For this review, take the finished solid that the model builds, in its own axes (mm). Face numbers are marked on the shaded views. A direction names the side the tool comes from. Round coordinates to 2 decimals unless told otherwise and drop trailing zeros. Order: outer loops, then holes, each group sorted by start corner. A loop starts at its lowest first (then second) coordinate and runs counter-clockwise, first axis right, second up. Notation, with made-up numbers: M 42,12.25 L 71,12.25 A25 ccw 71,33.25 Z; hole C 0.25,46 d1. An arc over 180 degrees is marked long. Answer as a JSON object with one key per item and string values.
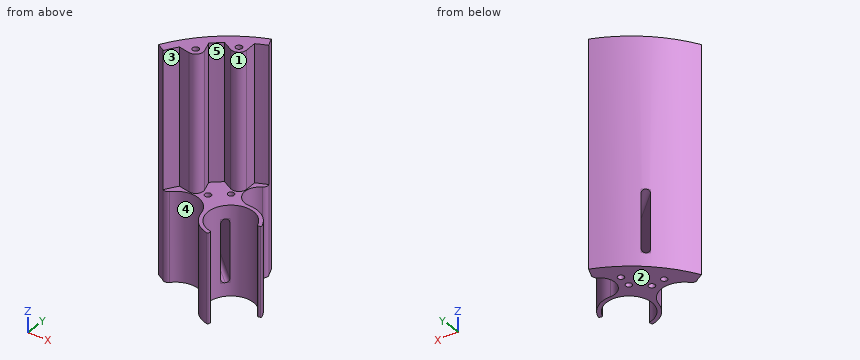
from build123d import *

# Parameters (mm, degrees)
BOSS_EXTRUDE1_DEPTH     = 119
BOSS_EXTRUDE2_DEPTH     = 47
SKETCH4_R               = 1.65
CUT_EXTRUDE1_DEPTH      = 151.148950374
CUT_EXTRUDE2_START      = 44
CUT_EXTRUDE2_DEPTH      = 2.6
BOSS_EXTRUDE3_DEPTH     = 119
SKETCH7_R               = 1.65
CUT_EXTRUDE3_DEPTH      = 151.148950374
CUT_EXTRUDE4_START      = 116
CUT_EXTRUDE4_DEPTH      = 2.6
CUT_EXTRUDE5_START      = 3
CUT_EXTRUDE5_DEPTH      = 2.6
CUT_EXTRUDE_THIN1_DEPTH = 151.148950374
CUT_EXTRUDE6_START      = 7
CUT_EXTRUDE6_DEPTH      = 33
FILLET1_R               = 2


with BuildPart() as part:
    # Sketch1 → Boss-Extrude1 (new body)
    with BuildSketch(Plane(origin=(0, 0, 0), x_dir=(0, 1, 0), z_dir=(0, 0, 1))):
        with BuildLine():
            Line((66.793011614, 25.63943495), (62.125109481, 23.847595202))
            ThreePointArc((62.125109481, 23.847595202), (50.18784505, 43.696878999), (32.170193606, 58.252173078))
            Line((32.170193606, 58.252173078), (34.587369472, 62.629073903))
            ThreePointArc((34.587369472, 62.629073903), (53.95881545, 46.980136869), (66.793011614, 25.63943495))
        make_face()
    extrude(amount=BOSS_EXTRUDE1_DEPTH)

    # Sketch3 → Boss-Extrude2 (add)
    with BuildSketch(Plane(origin=(0, 0, 0), x_dir=(0, 1, 0), z_dir=(0, 0, 1))):
        with BuildLine():
            Line((16.662914887, 22.849921086), (17.643603591, 22.654345869))
            ThreePointArc((17.643603591, 22.654345869), (18.018970735, 22.728818123), (18.231735551, 23.046902612))
            ThreePointArc((18.231735551, 23.046902612), (37.916609506, 29.718164665), (33.851654942, 9.334932723))
            ThreePointArc((33.851654942, 9.334932723), (33.563813587, 9.082754287), (33.538596095, 8.700902631))
            Line((33.538596095, 8.700902631), (33.85956734, 7.753813691))
            ThreePointArc((33.85956734, 7.753813691), (34.111745776, 7.465972336), (34.493597433, 7.440754844))
            ThreePointArc((34.493597433, 7.440754844), (41.448499021, 12.641968592), (43.997873295, 20.944014808))
            ThreePointArc((43.997873295, 20.944014808), (49.930251766, 28.811968202), (58.997685125, 24.954578252))
            ThreePointArc((58.997685125, 24.954578252), (60.351321071, 23.807583941), (62.125109481, 23.847595202))
            ThreePointArc((62.125109481, 23.847595202), (50.18784505, 43.696878999), (32.170193606, 58.252173078))
            ThreePointArc((32.170193606, 58.252173078), (31.867825608, 56.602303211), (32.676329677, 55.132671232))
            ThreePointArc((32.676329677, 55.132671232), (36.307290349, 43.066223982), (27.152640183, 34.407390053))
            ThreePointArc((27.152640183, 34.407390053), (20.061145201, 30.559977956), (16.270358143, 23.438053047))
            ThreePointArc((16.270358143, 23.438053047), (16.344830398, 23.062685903), (16.662914887, 22.849921086))
        make_face()
    extrude(amount=BOSS_EXTRUDE2_DEPTH)

    # Sketch4 → Cut-Extrude1 (cut, through all)
    with BuildSketch(Plane(origin=(0, 0, 0), x_dir=(0, 1, 0), z_dir=(0, 0, 1))):
        with Locations(Location((40.305086528, 40.305086528, 0), (0, 0, 270))):
            Circle(SKETCH4_R)
        with Locations(Location((46.691666524, 32.693856872, 0), (0, 0, 270))):
            Circle(SKETCH4_R)
    extrude(amount=CUT_EXTRUDE1_DEPTH, mode=Mode.SUBTRACT)

    # Sketch5 → Cut-Extrude2 (cut)
    with BuildSketch(Plane(origin=(0, 0, 0), x_dir=(0, 1, 0), z_dir=(0, 0, 1)).offset(CUT_EXTRUDE2_START)):
        Polygon((43.480513008, 40.305086528), (41.892799768, 43.055086528), (38.717373287, 43.055086528), (37.129660047, 40.305086528), (38.717373287, 37.555086528), (41.892799768, 37.555086528), align=None)
        Polygon((49.867093005, 32.693856872), (48.279379765, 35.443856872), (45.103953284, 35.443856872), (43.516240044, 32.693856872), (45.103953284, 29.943856872), (48.279379765, 29.943856872), align=None)
    extrude(amount=-CUT_EXTRUDE2_DEPTH, mode=Mode.SUBTRACT)

    # Sketch6 → Boss-Extrude3 (add)
    with BuildSketch(Plane(origin=(0, 0, 0), x_dir=(0, 1, 0), z_dir=(0, 0, 1))):
        with BuildLine():
            ThreePointArc((38.577322779, 54.222017596), (43.657448084, 50.222149016), (48.32540701, 45.748137255))
            Line((48.32540701, 45.748137255), (42.663514101, 43.798591183))
            ThreePointArc((42.663514101, 43.798591183), (38.737005367, 44.561827164), (37.434732749, 48.343901467))
            Line((37.434732749, 48.343901467), (38.577322779, 54.222017596))
        make_face()
        with BuildLine():
            ThreePointArc((52.744660964, 40.57385568), (56.433360559, 35.263477438), (59.589277435, 29.620179604))
            Line((59.589277435, 29.620179604), (53.604790209, 29.411196706))
            ThreePointArc((53.604790209, 29.411196706), (50.072999838, 31.289082957), (49.933401851, 35.286646265))
            Line((49.933401851, 35.286646265), (52.744660964, 40.57385568))
        make_face()
    extrude(amount=BOSS_EXTRUDE3_DEPTH)

    # Sketch7 → Cut-Extrude3 (cut, through all)
    with BuildSketch(Plane(origin=(0, 0, 0), x_dir=(0, 1, 0), z_dir=(0, 0, 1))):
        with Locations(Location((41.361241483, 47.580665485, 0), (0, 0, 270))):
            Circle(SKETCH7_R)
        with Locations(Location((53.465192222, 33.408760014, 0), (0, 0, 270))):
            Circle(SKETCH7_R)
    extrude(amount=CUT_EXTRUDE3_DEPTH, mode=Mode.SUBTRACT)

    # Sketch8 → Cut-Extrude4 (cut)
    with BuildSketch(Plane(origin=(0, 0, 0), x_dir=(0, 1, 0), z_dir=(0, 0, 1)).offset(CUT_EXTRUDE4_START)):
        Polygon((44.536667963, 47.580665485), (42.948954723, 50.330665485), (39.773528242, 50.330665485), (38.185815002, 47.580665485), (39.773528242, 44.830665485), (42.948954723, 44.830665485), align=None)
        Polygon((56.640618703, 33.408760014), (55.052905462, 36.158760014), (51.877478982, 36.158760014), (50.289765742, 33.408760014), (51.877478982, 30.658760014), (55.052905462, 30.658760014), align=None)
    extrude(amount=-CUT_EXTRUDE4_DEPTH, mode=Mode.SUBTRACT)

    # Sketch5<2> → Cut-Extrude5 (cut)
    with BuildSketch(Plane(origin=(0, 0, 0), x_dir=(0, 1, 0), z_dir=(0, 0, 1)).offset(CUT_EXTRUDE5_START)):
        Polygon((43.480513008, 40.305086528), (41.892799768, 43.055086528), (38.717373287, 43.055086528), (37.129660047, 40.305086528), (38.717373287, 37.555086528), (41.892799768, 37.555086528), align=None)
        Polygon((49.867093005, 32.693856872), (48.279379765, 35.443856872), (45.103953284, 35.443856872), (43.516240044, 32.693856872), (45.103953284, 29.943856872), (48.279379765, 29.943856872), align=None)
    extrude(amount=CUT_EXTRUDE5_DEPTH, mode=Mode.SUBTRACT)

    # Sketch9 → Cut-Extrude-Thin1 (cut, through all)
    with BuildSketch(Plane(origin=(0, 0, 0), x_dir=(0, 1, 0), z_dir=(0, 0, 1))):
        Polygon((62.178864674, 23.707558139), (66.846766806, 25.499397886), (66.739256421, 25.779472014), (62.071354289, 23.987632266), align=None)
        Polygon((32.301500631, 58.179657802), (34.718676497, 62.556558627), (34.456062447, 62.701589179), (32.038886581, 58.324688354), align=None)
    extrude(amount=CUT_EXTRUDE_THIN1_DEPTH, mode=Mode.SUBTRACT)

    # Sketch10 → Cut-Extrude6 (cut)
    with BuildSketch(Plane(origin=(0, 0, 0), x_dir=(0, 1, 0), z_dir=(0, 0, 1)).offset(CUT_EXTRUDE6_START)):
        Polygon((35.44701831, 29.64338025), (54.282655982, 50.303964956), (57.23861856, 47.609102207), (38.402980888, 26.948517501), align=None)
    extrude(amount=CUT_EXTRUDE6_DEPTH, mode=Mode.SUBTRACT)

    # Fillet1
    # the kernel refuses this fillet: 2 mm, written as the material it adds along each edge
    with BuildSketch(Plane(origin=(-27.096333376, 33.124951788, 40), x_dir=(0.673715687259404, 0.7389906445555241, 0), z_dir=(-0.7389906445555242, 0.673715687259404, 0))) as fillet1_piece_1_section:
        with BuildLine():
            CenterArc((FILLET1_R, FILLET1_R), FILLET1_R, 180, 90)
            Line((0, FILLET1_R), (0, 0))
            Line((0, 0), (FILLET1_R, 0))
        make_face()
    fillet1_piece_1 = extrude(amount=33.933040427, mode=Mode.PRIVATE)
    fillet1_piece_1 = fillet1_piece_1 & Plane(origin=(0, 0, 39.546220167), x_dir=(-0.8753801649783101, 0.4834351732782244, 0), z_dir=(0, 0, -1)) * Cylinder(71.545, 76, mode=Mode.PRIVATE)
    fillet1_piece_1 = fillet1_piece_1 - Plane(origin=(-20.7, 30, 39.546220167), x_dir=(-0.19557521764305516, -0.9806887040462288, 0), z_dir=(0, 0, -1)) * Cylinder(12, 76, mode=Mode.PRIVATE)
    add(fillet1_piece_1)
    with BuildSketch(Plane(origin=(-49.13548978, 58.630180498, 40), x_dir=(-0.6737156872594037, -0.7389906445555243, 0), z_dir=(0.7389906445555244, -0.6737156872594038, 0))) as fillet1_piece_2_section:
        with BuildLine():
            CenterArc((FILLET1_R, FILLET1_R), FILLET1_R, 180, 90)
            Line((0, FILLET1_R), (0, 0))
            Line((0, 0), (FILLET1_R, 0))
        make_face()
    fillet1_piece_2 = extrude(amount=33.470003085, mode=Mode.PRIVATE)
    fillet1_piece_2 = fillet1_piece_2 & Plane(origin=(0, 0, 39.547293042), x_dir=(-0.8753801649783101, 0.4834351732782244, 0), z_dir=(0, 0, -1)) * Cylinder(71.545, 75, mode=Mode.PRIVATE)
    fillet1_piece_2 = fillet1_piece_2 - Plane(origin=(-20.7, 30, 39.547293042), x_dir=(-0.19557521764305516, -0.9806887040462288, 0), z_dir=(0, 0, -1)) * Cylinder(12, 75, mode=Mode.PRIVATE)
    add(fillet1_piece_2)
    with BuildSketch(Plane(origin=(-27.096333376, 33.124951788, 7), x_dir=(0.673715687259404, 0.7389906445555241, 0), z_dir=(-0.7389906445555242, 0.673715687259404, 0))) as fillet1_piece_3_section:
        with BuildLine():
            CenterArc((FILLET1_R, -FILLET1_R), FILLET1_R, 90, 90)
            Line((0, -FILLET1_R), (0, 0))
            Line((0, 0), (FILLET1_R, 0))
        make_face()
    fillet1_piece_3 = extrude(amount=33.933040427, mode=Mode.PRIVATE)
    fillet1_piece_3 = fillet1_piece_3 & Plane(origin=(0, 0, 7.453779833), x_dir=(-0.8753801649783101, 0.4834351732782244, 0), z_dir=(0, 0, -1)) * Cylinder(71.545, 76, mode=Mode.PRIVATE)
    fillet1_piece_3 = fillet1_piece_3 - Plane(origin=(-20.7, 30, 7.453779833), x_dir=(-0.19557521764305516, -0.9806887040462288, 0), z_dir=(0, 0, -1)) * Cylinder(12, 76, mode=Mode.PRIVATE)
    add(fillet1_piece_3)
    with BuildSketch(Plane(origin=(-49.13548978, 58.630180498, 7), x_dir=(0, 0, 1), z_dir=(0.7389906445555244, -0.6737156872594038, 0))) as fillet1_piece_4_section:
        with BuildLine():
            CenterArc((FILLET1_R, FILLET1_R), FILLET1_R, 180, 90)
            Line((0, FILLET1_R), (0, 0))
            Line((0, 0), (FILLET1_R, 0))
        make_face()
    fillet1_piece_4 = extrude(amount=33.470003085, mode=Mode.PRIVATE)
    fillet1_piece_4 = fillet1_piece_4 & Plane(origin=(0, 0, 7.452710361), x_dir=(-0.8753801649783101, 0.4834351732782244, 0), z_dir=(0, 0, -1)) * Cylinder(71.545, 75, mode=Mode.PRIVATE)
    fillet1_piece_4 = fillet1_piece_4 - Plane(origin=(-20.7, 30, 7.452710361), x_dir=(-0.19557521764305516, -0.9806887040462288, 0), z_dir=(0, 0, -1)) * Cylinder(12, 75, mode=Mode.PRIVATE)
    add(fillet1_piece_4)


solid = part.part
1) For L1, parallel to X at y = 40, z = 19.5; L2, parallel to Y at x = -44.5, z = 31; L3, parallel to Z at x = -32.5, y = 34, list the stretches that pass through material, from the lowest coordinate up.
Geometry check:
{"L1": "x = -59.32 to -48.51, -46.65 to -41.93, -38.68 to -34.64, -28.7 to -27.33, -14.07 to -10.9", "L2": "y = 36.6 to 48.99, 54.4 to 56.02", "L3": "z = 0 to 47"}
2) Mouldability with a two-part tool opening along X and no side actions: class the marked faces 1 and 2 as +X half, -X half, draft (parallel to the pull), parting line (faces both ways), or undercut.
Geometry check:
{"face 1": "undercut", "face 2": "draft"}
3) Insertion check: P1, Ø1, axis at y = 41, z = 63, coming from the -X side; P2, Ø3, axis at y = 53, z = 115, coming from the +X side; P3, Ø2, axis at y = 35.5, z = 19.5, coming from the +X side; P4, Ø1.7, axis at x = -34.5, y = 54.5, coming from the -Z side. Each pin has a flat end and moves straight along its axis. Give the tip position at first contact, or say it passes through.
Geometry check:
{"P1": "stops at x = -58.98", "P2": "stops at x = -29.41", "P3": "stops at x = -7.44", "P4": "stops at z = 0"}
4) Machinability: for the marked faces 3, 4 and 5, which of the approach directions +Z, -Z, +X, -X, +Y, -Y give a long, thin tool a straight path to every point of the face, cutting with its end or side? Answer none if there is none.
Geometry check:
{"face 3": "+Z, -Y", "face 4": "+Z, -Z, -Y", "face 5": "+Z"}
5) Add section C-C on x = -13.5. State the section outline as (y, z) points, and give its area (3 significant figures).
Geometry check:
{"outline": "M 39.6,0 L 42.01,0 L 42.01,47 L 39.6,47 Z", "area": "113 mm²"}
6) Add section D-D on y = 29.5. State the section outline as (x, z) points, and give its area (3 significant figures).
Geometry check:
{"outline": "M -35.15,0 L -32.69,0 L -32.69,47 L -35.15,47 Z", "area": "116 mm²"}
7) Add section A-A on z = 29. State how many separate pieces and enclosed holes the cut face has, and give its area (3 significant figures).
Geometry check:
{"separate pieces": "2", "enclosed holes": "4", "area": "662 mm²"}
